```python
from build123d import *

# Parameters (mm, degrees)
F0_R      = 3
F1_DEPTH  = 5
F2_DEPTH  = 5
F3_R      = 5
F4_R      = 5
F5_DEPTH  = 2
F6_DEPTH  = 2
F7_DEPTH  = 2
F8_DEPTH  = 2
F9_DEPTH  = 2
F10_DEPTH = 2
F11_R     = 5


with BuildPart() as f1:
    # F0 (on Top) → F1 (new body)
    with BuildSketch(Plane.XY):
        Polygon((-60.669873, 115.083302), (-65, 112.583302), (-69.330127, 110.083302), (-130, 5), (-130, 0), (-130, -5), (-69.330127, -110.083302), (-65, -112.583302), (-60.669873, -115.083302), (60.669873, -115.083302), (65, -112.583302), (69.330127, -110.083302), (130, -5), (130, 0), (130, 5), (69.330127, 110.083302), (65, 112.583302), (60.669873, 115.083302), align=None)
        with Locations((-62.5, -108.253175)):
            Circle(F0_R, mode=Mode.SUBTRACT)
        with Locations((-125, 0)):
            Circle(F0_R, mode=Mode.SUBTRACT)
        with Locations((62.5, -108.253175)):
            Circle(F0_R, mode=Mode.SUBTRACT)
        Polygon((64.330127, 101.423048), (120, 5), (120, -5), (64.330127, -101.423048), (55.669873, -106.423048), (-55.669873, -106.423048), (-64.330127, -101.423048), (-120, -5), (-120, 5), (-64.330127, 101.423048), (-60, 103.923048), (-55.669873, 106.423048), (55.669873, 106.423048), (60, 103.923048), align=None, mode=Mode.SUBTRACT)
        with Locations((125, 0)):
            Circle(F0_R, mode=Mode.SUBTRACT)
        with Locations((-62.5, 108.253175)):
            Circle(F0_R, mode=Mode.SUBTRACT)
        with Locations((62.5, 108.253175)):
            Circle(F0_R, mode=Mode.SUBTRACT)
    extrude(amount=F1_DEPTH)

    # F0 (on Top) → F2 (join)
    with BuildSketch(Plane.XY):
        with BuildLine():
            ThreePointArc((19.364917, -5), (19.840594, -2.520086), (20, 0))
            ThreePointArc((20, 0), (19.840594, 2.520086), (19.364917, 5))
            ThreePointArc((19.364917, 5), (17.320508, 10), (14.012585, 14.27051))
            ThreePointArc((14.012585, 14.27051), (10, 17.320508), (5.352331, 19.27051))
            ThreePointArc((5.352331, 19.27051), (0, 20), (-5.352331, 19.27051))
            ThreePointArc((-5.352331, 19.27051), (-10, 17.320508), (-14.012585, 14.27051))
            ThreePointArc((-14.012585, 14.27051), (-17.320508, 10), (-19.364917, 5))
            ThreePointArc((-19.364917, 5), (-20, 0), (-19.364917, -5))
            ThreePointArc((-19.364917, -5), (-17.320508, -10), (-14.012585, -14.27051))
            ThreePointArc((-14.012585, -14.27051), (-10, -17.320508), (-5.352331, -19.27051))
            ThreePointArc((-5.352331, -19.27051), (0, -20), (5.352331, -19.27051))
            ThreePointArc((5.352331, -19.27051), (10, -17.320508), (14.012585, -14.27051))
            ThreePointArc((14.012585, -14.27051), (17.320508, -10), (19.364917, -5))
        make_face()
        with BuildLine():
            ThreePointArc((-19.364917, -5), (-20, 0), (-19.364917, 5))
            Line((-19.364917, 5), (-120, 5))
            Line((-120, 5), (-120, -5))
            Line((-120, -5), (-19.364917, -5))
        make_face()
        with BuildLine():
            ThreePointArc((-14.012585, 14.27051), (-10, 17.320508), (-5.352331, 19.27051))
            Line((-5.352331, 19.27051), (-55.669873, 106.423048))
            Line((-55.669873, 106.423048), (-60, 103.923048))
            Line((-60, 103.923048), (-64.330127, 101.423048))
            Line((-64.330127, 101.423048), (-14.012585, 14.27051))
        make_face()
        with BuildLine():
            ThreePointArc((5.352331, 19.27051), (10, 17.320508), (14.012585, 14.27051))
            Line((14.012585, 14.27051), (64.330127, 101.423048))
            Line((64.330127, 101.423048), (60, 103.923048))
            Line((60, 103.923048), (55.669873, 106.423048))
            Line((55.669873, 106.423048), (5.352331, 19.27051))
        make_face()
        with BuildLine():
            ThreePointArc((19.364917, 5), (19.840594, 2.520086), (20, 0))
            ThreePointArc((20, 0), (19.840594, -2.520086), (19.364917, -5))
            Line((19.364917, -5), (120, -5))
            Line((120, -5), (120, 5))
            Line((120, 5), (19.364917, 5))
        make_face()
        with BuildLine():
            Line((64.330127, -101.423048), (14.012585, -14.27051))
            ThreePointArc((14.012585, -14.27051), (10, -17.320508), (5.352331, -19.27051))
            Line((5.352331, -19.27051), (55.669873, -106.423048))
            Line((55.669873, -106.423048), (64.330127, -101.423048))
        make_face()
        with BuildLine():
            Line((-55.669873, -106.423048), (-5.352331, -19.27051))
            ThreePointArc((-5.352331, -19.27051), (-10, -17.320508), (-14.012585, -14.27051))
            Line((-14.012585, -14.27051), (-64.330127, -101.423048))
            Line((-64.330127, -101.423048), (-55.669873, -106.423048))
        make_face()
    extrude(amount=F2_DEPTH)

    # F3
    f3_edges = [f1.edges().sort_by_distance(p)[0] for p in [
        (-60.669873, -115.083302, 2.5),
    ]]
    fillet(f3_edges, radius=F3_R)

    # F4
    f4_edges = [f1.edges().sort_by_distance(p)[0] for p in [
        (-69.330127, -110.083302, 2.5),
        (60.669873, -115.083302, 2.5),
        (69.330127, -110.083302, 2.5),
        (130, -5, 2.5),
        (130, 5, 2.5),
        (69.330127, 110.083302, 2.5),
        (60.669873, 115.083302, 2.5),
        (-60.669873, 115.083302, 2.5),
        (-69.330127, 110.083302, 2.5),
        (-130, 5, 2.5),
        (-130, -5, 2.5),
    ]]
    fillet(f4_edges, radius=F4_R)

    # F0 (on Top) → F5 (join)
    with BuildSketch(Plane.XY):
        with Locations((-125, 0)):
            Circle(F0_R)
    extrude(amount=F5_DEPTH)

    # F0 (on Top) → F6 (join)
    with BuildSketch(Plane.XY):
        with Locations((-62.5, 108.253175)):
            Circle(F0_R)
    extrude(amount=F6_DEPTH)

    # F0 (on Top) → F7 (join)
    with BuildSketch(Plane.XY):
        with Locations((62.5, 108.253175)):
            Circle(F0_R)
    extrude(amount=F7_DEPTH)

    # F0 (on Top) → F8 (join)
    with BuildSketch(Plane.XY):
        with Locations((125, 0)):
            Circle(F0_R)
    extrude(amount=F8_DEPTH)

    # F0 (on Top) → F9 (join)
    with BuildSketch(Plane.XY):
        with Locations((62.5, -108.253175)):
            Circle(F0_R)
    extrude(amount=F9_DEPTH)

    # F0 (on Top) → F10 (join)
    with BuildSketch(Plane.XY):
        with Locations((-62.5, -108.253175)):
            Circle(F0_R)
    extrude(amount=F10_DEPTH)

    # F11
    f11_edges = [f1.edges().sort_by_distance(p)[0] for p in [
        (-64.330127, -101.423048, 2.5),
        (-120, -5, 2.5),
        (-120, 5, 2.5),
        (-64.330127, 101.423048, 2.5),
        (-55.669873, 106.423048, 2.5),
        (55.669873, 106.423048, 2.5),
        (64.330127, 101.423048, 2.5),
        (120, 5, 2.5),
        (120, -5, 2.5),
        (64.330127, -101.423048, 2.5),
        (55.669873, -106.423048, 2.5),
        (-55.669873, -106.423048, 2.5),
    ]]
    fillet(f11_edges, radius=F11_R)


solid = f1.part
```
For this review, take the finished solid that the model builds, in its own axes (mm). A direction names the side the tool comes from. Coordinates: 2 decimals unless noted, no trailing zeros. Order: outer loops, then holes, each group sorted by start corner. A loop starts at its lowest first (then second) coordinate and runs counter-clockwise, first axis right, second up. Notation, with made-up numbers: (-5.75, 50.25) -> (2.25, 50.25) arc R10 cw to (2.25, 66.25) -> close; hole circle Ø9 at (64.5, -28.5). An arc over 180 degrees is marked (long way). Use CSV: the item, a comma, the result in double quotes. Start each with the question number.
Item 1: For faces 5 (the face through (99.25, -58.26, 2.46)), 6 (the face through (-122.14, 0.9, 3.48)), 7 (the face through (92.494, -52.642, 2.465)), list the 3-axis set-ups (+Z, -Z, +X, -X, +Y, -Y) from which the entire face can be reached by the end or side of a thin tool; tool diameter is ignored.
Item 2: We need section C-C, the plane y = 54. Give the boundary of the cut face in (x, z).
Item 3: Wall thickness on probe 1 along X at (y, z) = (-43, 4); probe 2 along Y at (x, z) = (-62.5, 3.85); probe 3 along X at (y, z) = (37.5, 1.25): over which ranges is each line inside the solid? List them lowest first.
Item 4: Draft analysis for pull direction Y (two halves, no side actions). For faces 1 (the face through (-1, 1, 0)), 2 (the face through (-17.28, 10.07, 2.46)), 3 (the face through (62, 108, 2)), 4 (the face through (-99.25, 58.26, 2.46)), state which applies: pulls with the +Y half, pulls with the -Y half, needs draft (parallel to the pull), parting line crosses it, or undercut.
Item 5: We need section D-D, the plane z = 4.15. Give the number of separate pieces and of enclosed holes in the cut face, then the cut area to 3 significant figures.
Item 6: We need section B-B, the plane x = -108.5. Give the boundary of the cut face in (y, z), then the cut area to 3 significant figures.
Item 7: We need section A-A, the plane y = -9. Give the boundary of the cut face in (x, z), then the cut area to 3 significant figures.
Item 8: Insertion check: pin 1 (3 mm diameter, centred on y = -15.5, z = 4, fed in from +X); pin 2 (5 mm diameter, centred on x = 62.5, y = 108.25, fed in from +Z); pin 3 (3 mm diameter, centred on x = 99.5, z = 4, fed in from +Y). Each pin has a flat end and moves straight along its axis. Give the tip position at first contact, or say it passes through.
Derived:
1,face 5,"+Z, -Z, +X, -Y"
1,face 6,"+Z"
1,face 7,"+Z, -Z"
2,outline,"(-101.71, 0) -> (-91.71, 0) -> (-91.71, 5) -> (-101.71, 5) -> close; (-36.95, 0) -> (-25.4, 0) -> (-25.4, 5) -> (-36.95, 5) -> close; (25.4, 0) -> (36.95, 0) -> (36.95, 5) -> (25.4, 5) -> close; (91.71, 0) -> (101.71, 0) -> (101.71, 5) -> (91.71, 5) -> close"
3,probe 1,"x = -108.06 to -98.06, -30.6 to -19.05, 19.05 to 30.6, 98.06 to 108.06"
3,probe 2,"y = -114.03 to -111.25, -105.25 to -96.08, -5 to 5, 96.08 to 105.25, 111.25 to 114.03"
3,probe 3,"x = -111.24 to -101.24, -27.42 to -15.88, 15.88 to 27.42, 101.24 to 111.24"
4,face 1,"needs draft"
4,face 2,"undercut"
4,face 3,"undercut"
4,face 4,"pulls with the +Y half"
5,separate pieces,"1"
5,enclosed holes,"12"
5,area,"13,900 mm^2"
6,outline,"(-42.24, 0) -> (-24.92, 0) -> (-24.92, 5) -> (-42.24, 5) -> close; (-5, 0) -> (5, 0) -> (5, 5) -> (-5, 5) -> close; (24.92, 0) -> (42.24, 0) -> (42.24, 5) -> (24.92, 5) -> close"
6,area,"223 mm^2"
7,outline,"(-127.69, 0) -> (-116.24, 0) -> (-116.24, 5) -> (-127.69, 5) -> close; (-17.86, 0) -> (17.86, 0) -> (17.86, 5) -> (-17.86, 5) -> close; (116.24, 0) -> (127.69, 0) -> (127.69, 5) -> (116.24, 5) -> close"
7,area,"293 mm^2"
8,pin 1,"stops at x = 124.8"
8,pin 2,"stops at z = 2"
8,pin 3,"stops at y = 60.43"
